Input: dimensioned drawing with shaded views. Units: mm. Origin: part minimum x, y, z. A direction names the side the tool comes from. Give positions to 0.01 mm unless a question says otherwise; leave off trailing zeros. Write each loop counter-clockwise with the first axis right and the second up, starting at its lowest first coordinate (ties: lowest second). Pieces come first, ordered by that corner, then holes. Notation, with made-up numbers: M 37,25.25 L 51,25.25 A4 ccw 51,31.25 Z; hole C 67.5,70 d5. An arc over 180 degrees is marked long. Use CSV: the item, a comma, the result in double quotes. Start each with the question number.
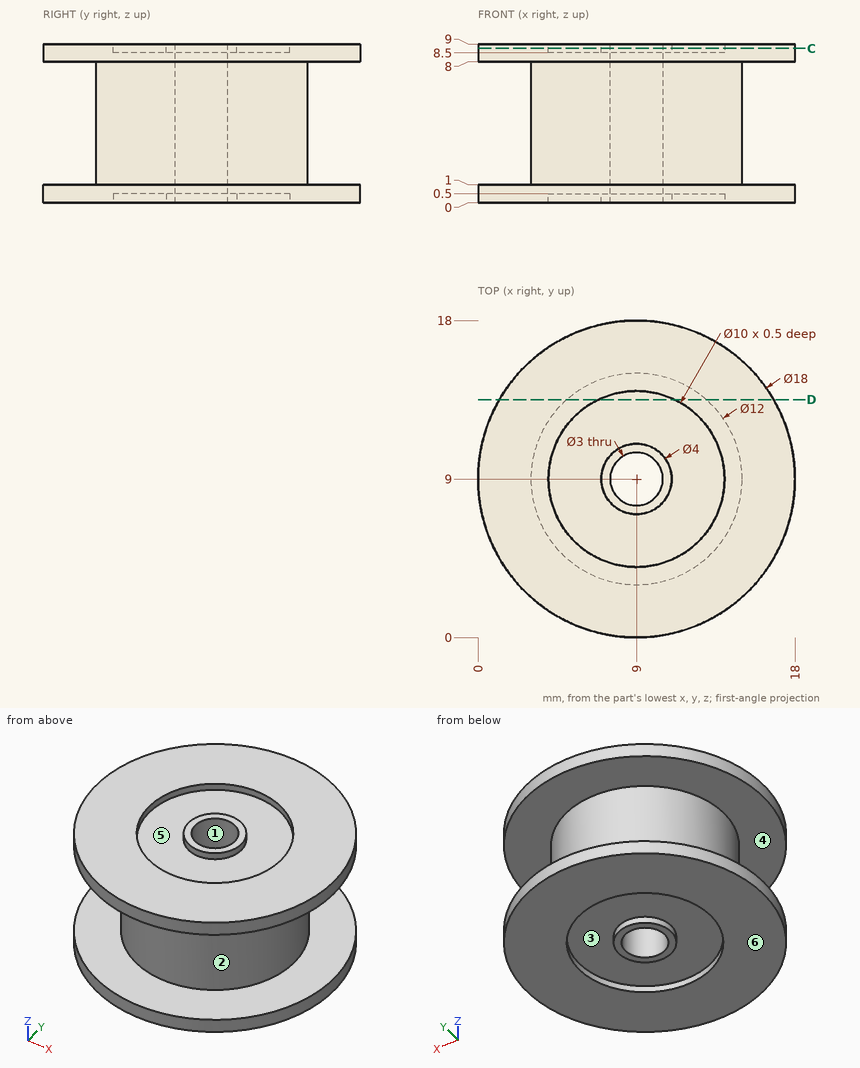
Q1. Material intervals for L1, parallel to Y at x = 9, z = 0.15; L2, parallel to Z at x = 6, y = 17; L3, parallel to Y at x = 9, z = 4, sorted ascending. Write a range as [from, to].
Q2. Set-up query: the marked faces 1, 2 and 3. Return all of +Z, -Z, +X, -X, +Y, -Y with unobstructed straight access to the full face (end or side cutting, diameter ignored); none if empty.
Q3. Pull-direction query (Z, two-part tool) for the marked faces 4, 5 and 6; classes: released by +Z, released by -Z, zero draft, split by the parting line, or undercut.
Q4. Section C-C, the plane z = 8.75. Return the cut outline in (x, y), and give its area (3 significant figures).
Q5. First-contact query: pin 1 Ø3 at (y, z) = (3.5, 8) entering from +X; pin 2 Ø2 at (y, z) = (10.5, 7.5) entering from +X; pin 3 Ø2 at (x, z) = (7.5, 1.5) entering from -Y; pin 4 Ø2.5 at (x, y) = (9, 9) entering from +Z. Flat tips, straight axial feed; report the tip coordinate or a pass-through.
Q6. Section D-D, the plane y = 13.5. Return the cut outline in (x, z).
Check result:
1,L1,"y = [0, 4], [7, 7.5], [10.5, 11], [14, 18]"
1,L2,"z = [0, 1], [8, 9]"
1,L3,"y = [3, 7.5], [10.5, 15]"
2,face 1,"+Z, -Z"
2,face 2,"none"
2,face 3,"-Z"
3,face 4,"undercut"
3,face 5,"released by +Z"
3,face 6,"released by -Z"
4,outline,"C 9,9 d18; C 9,9 d4; hole C 9,9 d10; hole C 9,9 d3"
4,area,"181 mm²"
5,pin 1,"stops at x = 17.06"
5,pin 2,"stops at x = 17.98"
5,pin 3,"stops at y = 0.02"
5,pin 4,"passes through"
6,outline,"M 1.21,0 L 6.82,0 L 6.82,0.5 L 11.18,0.5 L 11.18,0 L 16.79,0 L 16.79,1 L 12.97,1 L 12.97,8 L 16.79,8 L 16.79,9 L 11.18,9 L 11.18,8.5 L 6.82,8.5 L 6.82,9 L 1.21,9 L 1.21,8 L 5.03,8 L 5.03,1 L 1.21,1 Z"
